```python
from build123d import *

# Parameters (mm, degrees)
SKETCH1_W                = 6.8
SKETCH1_H                = 5
BOSS_EXTRUDE1_DEPTH      = 3.8
HOLE1_D                  = 1.05
HOLE1_CBORE_D            = 1.3
HOLE1_CBORE_DEPTH        = 1.2
CUT_EXTRUDE8_DEPTH       = 10.340235543
SKETCH20_W               = 5
SKETCH20_H               = 1.3
CUT_EXTRUDE11_DEPTH      = 0.3
M1_0X0_25_TAPPED_HOLE1_D = 0.75


with BuildPart() as part:
    # Sketch1 → Boss-Extrude1 (new body)
    with BuildSketch(Plane(origin=(0, 4, 0), x_dir=(-1, 0, 0), z_dir=(0, 1, 0))):
        with Locations((-3.4, 2.5)):
            Rectangle(SKETCH1_W, SKETCH1_H)
    extrude(amount=-BOSS_EXTRUDE1_DEPTH)

    # Hole1 (through all)
    with Locations(Plane(origin=(0, 0, 0), x_dir=(-1, 0, 0), z_dir=(0, 0, -1))):
        with Locations((-5.7, 1.7), (-0.7, 1.7)):
            CounterBoreHole(HOLE1_D / 2, HOLE1_CBORE_D / 2, HOLE1_CBORE_DEPTH)

    # Sketch17 → Cut-Extrude8 (cut, through all)
    with BuildSketch(Plane.XY.offset(5)):
        with BuildLine():
            Line((6.8, 2.225), (5.7, 2.225))
            ThreePointArc((5.7, 2.225), (6.07123106, 2.07123106), (6.225, 1.7))
            ThreePointArc((6.225, 1.7), (6.07123106, 1.32876894), (5.7, 1.175))
            Line((5.7, 1.175), (6.8, 1.175))
            Line((6.8, 1.175), (6.8, 2.225))
        make_face()
        with BuildLine():
            ThreePointArc((6.225, 1.7), (6.07123106, 2.07123106), (5.7, 2.225))
            Line((5.7, 2.225), (5.7, 1.175))
            ThreePointArc((5.7, 1.175), (6.07123106, 1.32876894), (6.225, 1.7))
        make_face()
        with BuildLine():
            Line((5.7, 1.175), (5.7, 2.225))
            ThreePointArc((5.7, 2.225), (5.175, 1.7), (5.7, 1.175))
        make_face()
    extrude(amount=-CUT_EXTRUDE8_DEPTH, mode=Mode.SUBTRACT)

    # Sketch20 → Cut-Extrude11 (cut)
    with BuildSketch(Plane(origin=(6.8, 0, 0), x_dir=(0, 0, -1), z_dir=(1, 0, 0))):
        with Locations((-2.5, 3.35)):
            Rectangle(SKETCH20_W, SKETCH20_H)
    extrude(amount=-CUT_EXTRUDE11_DEPTH, mode=Mode.SUBTRACT)

    # M1.0x0.25 Tapped Hole1 (through all)
    with Locations(Plane(origin=(0, 0, 0), x_dir=(-1, 0, 0), z_dir=(0, 0, -1))):
        with Locations((-3.2, 1.7)):
            Hole(M1_0X0_25_TAPPED_HOLE1_D / 2)


solid = part.part
```
Work out the finished part from the listing and answer in its coordinate system (mm). A direction names the side the tool comes from. Coordinates: 2 decimals unless noted, no trailing zeros. Write each loop counter-clockwise with the first axis right and the second up, starting at its lowest first coordinate (ties: lowest second). Pieces come first, ordered by that corner, then holes. Notation, with made-up numbers: (22.25, 41.5) - (65.25, 41.5) arc R11 ccw to (65.25, 45.5) - close; hole circle Ø10 at (-2, -37.75). An arc over 180 degrees is marked (long way). Answer as a JSON object with one key per item and string values.
Q1. Which of the six approach directions +Z, -Z, +X, -X, +Y, -Y give full straight-line access (tool end or side, diameter ignored) to faces 1 (the flat face through (6, 1.175, 3)), 2 (the flat face through (3, 3, 0)), 3 (the cylindrical face through (5.05, 1.68, 0.59))?
Results list:
{"face 1": "+Z, -Z, +X", "face 2": "-Z, +X, -X, +Y, -Y", "face 3": "-Z"}
Q2. Find section D-D (x = 3.2). Write down the section's boundary in (y, z) (3 decimals).
Results list:
{"outline": "(0.2, 0) - (1.325, 0) - (1.325, 5) - (0.2, 5) - close; (2.075, 0) - (4, 0) - (4, 5) - (2.075, 5) - close"}
Q3. Consider L1, parallel to Y at x = 0.7, z = 2.5 (3 decimals); L2, parallel to X at y = 1.9, z = 2.75; L3, parallel to Y at x = 0.7, z = 0.8. Determine where each line is inside the solid, lowest interval first. Write a range as from..to.
Results list:
{"L1": "y = 0.2..1.175, 2.225..4", "L2": "x = 0..0.21, 1.19..2.88, 3.52..5.21", "L3": "y = 0.2..1.05, 2.35..4"}
Q4. Find section B-B (y = 1.7). Write down the section's boundary in (x, z) (3 decimals), plus the area to 3 significant figures.
Results list:
{"outline": "(0, 0) - (0.05, 0) - (0.05, 1.2) - (0.175, 1.2) - (0.175, 5) - (0, 5) - close; (1.225, 1.2) - (1.35, 1.2) - (1.35, 0) - (2.825, 0) - (2.825, 5) - (1.225, 5) - close; (3.575, 0) - (5.05, 0) - (5.05, 1.2) - (5.175, 1.2) - (5.175, 5) - (3.575, 5) - close", "area": "16.4 mm^2"}
Q5. For a pull along Y with two mould halves and no side action, classify faces 4 (the flat face through (6.5, 3, 3)), 5 (the flat face through (3, 0.2, 3)), 6 (the flat face through (6, 2.225, 3)) as pulls with the +Y half, pulls with the -Y half, needs draft (parallel to the pull), parting line crosses it, or undercut.
Results list:
{"face 4": "needs draft", "face 5": "pulls with the -Y half", "face 6": "undercut"}
Q6. Find section A-A (x = 0.7). Write down the section's boundary in (y, z) (3 decimals).
Results list:
{"outline": "(0.2, 0) - (1.05, 0) - (1.05, 1.2) - (1.175, 1.2) - (1.175, 5) - (0.2, 5) - close; (2.225, 1.2) - (2.35, 1.2) - (2.35, 0) - (4, 0) - (4, 5) - (2.225, 5) - close"}
Q7. Find section C-C (z = 1.75). Write down the section's boundary in (x, y) (3 decimals), plus the area to 3 significant figures.
Results list:
{"outline": "(0, 0.2) - (6.8, 0.2) - (6.8, 1.175) - (5.7, 1.175) arc R0.525 cw to (5.7, 2.225) - (6.8, 2.225) - (6.8, 2.7) - (6.5, 2.7) - (6.5, 4) - (0, 4) - close; hole circle Ø1.05 at (0.7, 1.7); hole circle Ø0.75 at (3.2, 1.7)", "area": "22.6 mm^2"}
Q8. Given pin 1 Ø0.6 at (y, z) = (3.5, 2) entering from +X; pin 2 Ø0.5 at (x, y) = (5.5, 2) entering from -Z; pin 3 Ø0.8 at (x, y) = (0.7, 1.7) entering from -Z, each flat-ended and moving along its own axis, determine where each tip first touches the part or whether it passes through.
Results list:
{"pin 1": "stops at x = 6.5", "pin 2": "stops at z = 1.2", "pin 3": "passes through"}
